Geometry: final body of the model. Coordinates: model frame, mm. Face numbers are marked on the shaded views. A direction names the side the tool comes from. Round coordinates to 2 decimals unless told otherwise and drop trailing zeros. Loops run counter-clockwise (first coordinate to the right, second up) from the corner with the lowest first, then second, coordinate; pieces in that order, holes last. Notation, with made-up numbers: (79.25, 25.5) - (131.25, 25.5) arc R19 ccw to (131.25, 44.5) - close; hole circle Ø5 at (7.25, 13.5). An arc over 180 degrees is marked (long way). Return JSON: item names as keys, results as strings. Group by question number.
1. Material intervals for probe 1 along Z at (x, y) = (0, 2.7) (3 decimals); probe 2 along Y at (x, z) = (-2.75, 14.5) (3 decimals); probe 3 along X at (y, z) = (-3, 13.25), sorted ascending.
2. Section C-C on y = 2.75. Return loops of the section in (x, z) (3 decimals).
3. Section D-D on y = 4.5. Return loops of the section in (x, z).
4. First-contact query: pin 1 Ø12 at (x, z) = (-6, 3) entering from +Y (3 decimals); pin 2 Ø5.5 at (x, y) = (-14, 0) entering from +Z; pin 3 Ø0.5 at (y, z) = (5.5, 3.5) entering from +X; pin 4 Ø5 at (y, z) = (-1.5, 13) entering from -X. Flat tips, straight axial feed; report the tip coordinate or a pass-through.
5. Draft query along Y for the marked faces 4, 5, 6 and 7. Return one class per face: +Y half, -Y half, draft (parallel to the pull), parting line (faces both ways), or undercut.
6. Section B-B on z = 18.5. Return loops of the section in (x, y) (3 decimals).
7. Set-up query: the marked faces 1, 2 and 3. Return all of +Z, -Z, +X, -X, +Y, -Y with unobstructed straight access to the full face (end or side cutting, diameter ignored); none if empty.
8. Section A-A on x = -5. Return loops of the section in (y, z) (3 decimals), and give its area (3 significant figures).
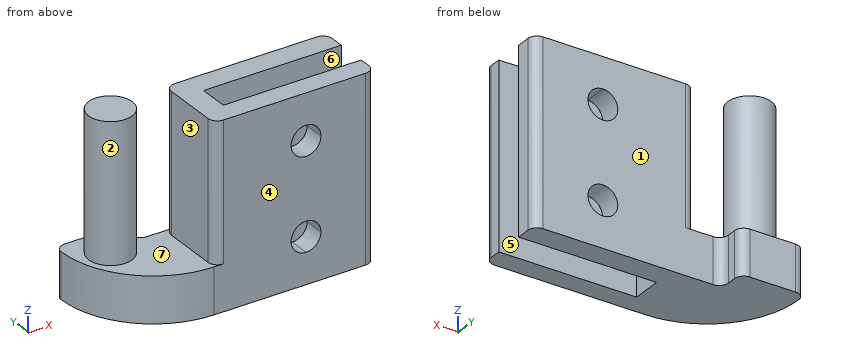
from build123d import *

# Parameters (mm, degrees)
F1_DEPTH = 20
F0_R     = 2.375
F2_DEPTH = 5
F3_DEPTH = 20
F4_R     = 1
F6_DEPTH = 8.5
F7_R     = 9.99999


# Not quite as in the source:
# - a fillet or chamfer is up to 0.001 mm smaller than in the source, because OpenCascade refuses the exact size


with BuildPart() as f1:
    # F0 (on Top) → F1 (new body)
    with BuildSketch(Plane.XY):
        Polygon((7.5, -3.875), (7.5, -1.625), (-7.5, -1.625), (-7.5, 1.625), (7.5, 1.625), (7.5, 4.125), (-10, 4.125), (-10, -3.875), align=None)
    extrude(amount=F1_DEPTH)

    # F0 (on Top) → F2 (join)
    with BuildSketch(Plane.XY):
        Polygon((-20, -3.875), (-10, -3.875), (-10, 4.125), (-13, 4.125), (-13, 7.125), (-20, 7.125), align=None)
        with Locations((-16.3791049272, 3.5122572444)):
            Circle(F0_R, mode=Mode.SUBTRACT)
    extrude(amount=F2_DEPTH)

    # F0 (on Top) → F3 (join)
    with BuildSketch(Plane.XY):
        with Locations((-16.3791049272, 3.5122572444)):
            Circle(F0_R)
    extrude(amount=F3_DEPTH)

    # F4
    f4_edges = [f1.edges().sort_by_distance(p)[0] for p in [
        (-20, 7.125, 2.5),
        (7.5, 4.125, 10),
        (7.5, -3.875, 10),
        (-10, 4.125, 12.5),
        (-10, -3.875, 12.5),
        (-13, 7.125, 2.5),
        (-13, 4.125, 2.5),
    ]]
    fillet(f4_edges, radius=F4_R)

    # F5 (on face) → F6 (cut)
    with BuildSketch(Plane.XZ.offset(3.875)):
        with BuildLine():
            ThreePointArc((1.625, 15), (1.1490485194, 16.1490485194), (0, 16.625))
            ThreePointArc((0, 16.625), (-1.1490485194, 13.8509514806), (1.625, 15))
        make_face()
        with BuildLine():
            ThreePointArc((1.625, 5), (-1.1490485194, 6.1490485194), (0, 3.375))
            ThreePointArc((0, 3.375), (1.1490485194, 3.8509514806), (1.625, 5))
        make_face()
    extrude(amount=-F6_DEPTH, mode=Mode.SUBTRACT)

    # F7 (radius 10 in the source; OpenCascade refuses exactly that, so slightly less here)
    f7_edges = [f1.edges().sort_by_distance(p)[0] for p in [
        (-20, -3.875, 2.5),
    ]]
    fillet(f7_edges, radius=F7_R)


solid = f1.part
Taken from the geometry:
{
 "1": {"probe 1": "0 to 3.375, 6.625 to 13.375, 16.625 to 20", "probe 2": "-3.875 to -1.625, 1.625 to 4.125", "probe 3": "-9.99 to 7.49"},
 "2": {"outline": "(-19.413, 0) - (7.5, 0) - (7.5, 20) - (-10, 20) - (-10, 5) - (-14.13, 5) - (-14.13, 20) - (-18.628, 20) - (-18.628, 5) - (-19.413, 5) - close; hole circle Ø3.25 at (0, 5); hole circle Ø3.25 at (0, 15)"},
 "3": {"outline": "(-19.87, 0) - (-12.78, 0) - (-12.78, 5) - (-14.22, 5) - (-14.22, 20) - (-18.54, 20) - (-18.54, 5) - (-19.87, 5) - close"},
 "4": {"pin 1": "y = 4.125", "pin 2": "z = 20", "pin 3": "x = -13", "pin 4": "x = -10"},
 "5": {"face 4": "-Y half", "face 5": "undercut", "face 6": "undercut", "face 7": "draft"},
 "6": {"outline": "circle Ø4.75 at (-16.379, 3.512); (-10, -2.875) arc R1 ccw to (-9, -3.875) - (6.5, -3.875) arc R1 ccw to (7.5, -2.875) - (7.5, -1.625) - (-7.5, -1.625) - (-7.5, 1.625) - (7.5, 1.625) - (7.5, 3.125) arc R1 ccw to (6.5, 4.125) - (-9, 4.125) arc R1 ccw to (-10, 3.125) - close"},
 "7": {"face 1": "+Z, -Z, +X, +Y", "face 2": "+Z", "face 3": "+Z, +Y, -Y"},
 "8": {"outline": "(-3.875, 0) - (-1.625, 0) - (-1.625, 20) - (-3.875, 20) - close; (1.625, 0) - (4.125, 0) - (4.125, 20) - (1.625, 20) - close", "area": "95.0 mm2"}
}
